Design review of the part built by this model. Coordinates are the model's own, in mm. A direction names the side the tool comes from. Coordinates: 2 decimals unless noted, no trailing zeros. Write each loop counter-clockwise with the first axis right and the second up, starting at its lowest first coordinate (ties: lowest second). Pieces come first, ordered by that corner, then holes.
Q1. For pin 1 Ø4 at (x, y) = (71, -2.5) entering from -Z; pin 2 Ø2 at (x, y) = (69, 0) entering from +Z, all flat-tipped, find the tip position at first contact; note any pin that passes through.
Q2. The part is to be moulded in two halves that separate along Y. For faces 1 (the flat face through (84.817, -1.382, 1.479)), 2 (the flat face through (79.816, 2.121, 1.479)), 3 (the flat face through (74.866, 2.828, 1.479)), say which applies: released by +Y, released by -Y, zero draft, split by the parting line, or undercut.
Q3. For L1, parallel to Y at x = 69, z = 0.8; L2, parallel to Y at x = 85.5, z = 2.4; L3, parallel to Y at x = 98, z = 2.8, list the stretches that pass through material, from the lowest coordinate up.
Q4. For faces 4 (the flat face through (79.867, -2.088, 1.479)), 5 (the flat face through (78, 0, 3)), list the 3-axis set-ups (+Z, -Z, +X, -X, +Y, -Y) from which the entire face can be reached by the end or side of a thin tool; tool diameter is ignored.
Q5. Take a section at A-A, the plane x = 69. Write out the cut boundary in (y, z), plus the area to 3 significant figures.
Autodesk Inventor part; units mm, degrees
ref_plane "YZ Plane" through (0, 0, 0) normal (1, 0, 0) x (0, 1, 0)
ref_plane "XZ Plane" through (0, 0, 0) normal (0, 1, 0) x (-1, 0, 0)
ref_plane "XY Plane" through (0, 0, 0) normal (0, 0, 1) x (1, 0, 0)
sketch "Sketch1" plane through (0, 0, 0) normal (0, 0, 1) x (1, 0, 0)
  spline S0 degree 4 poles (100, 0.032) (96.875, 0.4949) (92.5, 1.1413) (86.8751, 1.9754) (80.0002, 2.991) (75.0008, 3.7295) (70.0033, 4.4751) (65.0053, 5.1842) (60.0066, 5.8364) (55.0071, 6.4061) (50.0063, 6.8809) (45.0061, 7.2433) (40.0008, 7.4683) (35.0047, 7.533) (29.9791, 7.4197) (25.0319, 7.1346) (19.9582, 6.6428) (15.6359, 6.1039) (10.2184, 5.101) (7.8303, 4.4733) (5.3127, 3.8052) (2.8544, 2.7785) (1.5003, 2.0987) (0.6956, 1.3847) (0.5171, 1.2937) (-0.3402, 0) (0.5171, -1.2937) (0.6956, -1.3847) (1.5003, -2.0987) (2.8544, -2.7785) (5.3127, -3.8052) (7.8303, -4.4733) (10.2184, -5.101) (15.6359, -6.1039) (19.9582, -6.6428) (25.0319, -7.1346) (29.9791, -7.4197) (35.0047, -7.533) (40.0008, -7.4683) (45.0061, -7.2433) (50.0063, -6.8809) (55.0071, -6.4061) (60.0066, -5.8364) (65.0053, -5.1842) (70.0033, -4.4751) (75.0008, -3.7295) (80.0002, -2.991) (86.8751, -1.9754) (92.5, -1.1413) (96.875, -0.4949) (100, -0.032) knots 0 0 0 0 0 0.057355 0.080296 0.103238 0.126177 0.149108 0.172027 0.194928 0.217807 0.240666 0.263507 0.286336 0.309162 0.331999 0.354861 0.377772 0.399068 0.418771 0.436942 0.45243 0.465861 0.476678 0.486208 0.495579 0.504421 0.513792 0.523322 0.534139 0.54757 0.563058 0.581229 0.600932 0.622228 0.645139 0.668001 0.690838 0.713664 0.736493 0.759334 0.782193 0.805072 0.827973 0.850892 0.873823 0.896762 0.919704 0.942645 1 1 1 1 1
  circle A0 centre (26, 0) radius 2.5
  circle A1 centre (4, 0) radius 1.75
  circle A2 centre (69, 0) radius 1.75
  spline S1 degree 5 poles (8.9035, 0.2296) (9.2434, 0.8899) (11.3643, 2.0291) (18.2315, 3.5428) (20.2721, 2.9595) (23.0162, -3.0821) (16.5301, -2.3219) (12.7289, -2.0151) (9.2115, -1.112) (8.6356, -0.2907) (8.9035, 0.2296) knots 0 0 0 0 0 0 0.227523 0.364622 0.543771 0.698813 0.820709 1 1 1 1 1 1
  spline S2 degree 5 poles (31.2707, 2.5) (32.7339, 3.9218) (37.2285, 5.1212) (48.2817, 2.605) (61.2094, 6.6741) (64.3828, -5.6022) (45.0929, -1.179) (33.1446, -7.1128) (29.4849, -1.5962) (30.0097, 1.2748) (31.2707, 2.5) knots 0 0 0 0 0 0 0.215917 0.355077 0.532597 0.692902 0.813935 1 1 1 1 1 1
  line L0 (100, -0.032) -> (100.1, 0)
  line L1 (100.1, 0) -> (100, 0.032)
  circle A3 centre (69, 0) radius 4.5785
  line L2 (75, 3.731) -> (79.9461, 2.999)
  line L3 (79.9461, 2.999) -> (79.6826, 1.2184)
  line L4 (79.6826, 1.2184) -> (74.7365, 1.9504)
  line L5 (74.7365, 1.9504) -> (75, 3.731)
  line L6 (80, -2.991) -> (84.9463, -2.2599)
  line L7 (84.9463, -2.2599) -> (84.6831, -0.4793)
  line L8 (84.6831, -0.4793) -> (79.7368, -1.2103)
  line L9 (79.7368, -1.2103) -> (80, -2.991)
  point P0 (0, 0)
  point P1 (95, 0.772)
  point P2 (90, 1.512)
  point P3 (85, 2.252)
  point P4 (80, 2.991)
  point P5 (70, 4.468)
  point P6 (65, 5.173)
  point P7 (60, 5.82)
  point P8 (55, 6.387)
  point P9 (50, 6.858)
  point P10 (45, 7.215)
  point P11 (40, 7.435)
  point P12 (35, 7.496)
  point P13 (30, 7.384)
  point P14 (25, 7.091)
  point P15 (20, 6.619)
  point P16 (15, 5.942)
  point P17 (10, 4.997)
  point P18 (7.5, 4.382)
  point P19 (5, 3.618)
  point P20 (2.5, 2.579)
  point P21 (1.25, 1.844)
  point P22 (0.75, 1.448)
  point P23 (0.5, 1.203)
  point P24 (0, 0)
  point P25 (0.5, -1.203)
  point P26 (0.75, -1.448)
  point P27 (1.25, -1.844)
  point P28 (2.5, -2.579)
  point P29 (5, -3.618)
  point P30 (7.5, -4.382)
  point P31 (10, -4.997)
  point P32 (15, -5.942)
  point P33 (20, -6.619)
  point P34 (25, -7.091)
  point P35 (30, -7.384)
  point P36 (35, -7.496)
  point P37 (40, -7.435)
  point P38 (45, -7.215)
  point P39 (50, -6.858)
  point P40 (55, -6.387)
  point P41 (60, -5.82)
  point P42 (65, -5.173)
  point P43 (70, -4.468)
  point P44 (75, -3.731)
  point P45 (80, -2.991)
  point P46 (85, -2.252)
  point P47 (90, -1.512)
  point P48 (95, -0.772)
  point P49 (20.5674, 1.203)
  point P50 (21.0369, -1.512)
  point P51 (16.8986, -2.3616)
  point P52 (10, -1.1013)
  point P53 (59.6934, 1.7909)
  point P54 (60.4025, -1.203)
  point P55 (44.4534, -3.7857)
  point P56 (31.0165, -2.1426)
  point P57 (70, -4.468)
  point P58 (69.3082, 4.5682)
  point P59 (69.3082, -4.5682)
  dimension "d0" = 5
  dimension "d1" = 3.5
  dimension "d2" = 3.5
  dimension "d3" = 26
  dimension "d4" = 22
  dimension "d5" = 43
  dimension "d6" = 0.1
  dimension "d9" = 5
  dimension "d10" = 1.8
  dimension "d11" = 5
  dimension "d12" = 1.8
extrude "Extrusion1" add sketch "Sketch1" along normal blind 3 contours L1 L0 S0 L7 L8 L9 A3 L5 L4 L3 | A3 S0 picked at (65.4059, -0.3539)
properties part number "Tlotka"
Responses:
1. pin 1: stops at z = 0
1. pin 2: passes through
2. face 1: released by -Y
2. face 2: released by +Y
2. face 3: undercut
3. L1: y = -4.58 to -1.75, 1.75 to 4.58
3. L2: y = -2.18 to 2.18
3. L3: y = -0.33 to 0.33
4. face 4: +Z, -Z
4. face 5: +Z, +X, -X, +Y, -Y
5. outline: (-4.58, 0) - (-1.75, 0) - (-1.75, 3) - (-4.58, 3) - close; (1.75, 0) - (4.58, 0) - (4.58, 3) - (1.75, 3) - close
5. area: 17.0 mm2
